Check sheet for the modelled part. Datum: model origin and axes. Units: mm. Give positions to 0.01 mm unless a question says otherwise; leave off trailing zeros. Loops run counter-clockwise (first coordinate to the right, second up) from the corner with the lowest first, then second, coordinate; pieces in that order, holes last. Notation, with made-up numbers: (27.5, 54.5) -> (83.5, 54.5) arc R13 cw to (83.5, 59.5) -> close; hole circle Ø5 at (-36, -25.75). An arc over 180 degrees is marked (long way). Write each question's results on one line, items separated by ' | '. Start each with the question number.
Item 1: Cross-section at B-B on z = 1.4. Enter the section's corners in (x, y).
Item 2: Cross-section at C-C on x = -15. Enter the section's corners in (y, z).
Item 3: Cross-section at A-A on y = 19.5. Enter the section's corners in (x, z), then the cut area to 3 significant figures.
Item 4: Scan lines: line 1 along X through (y, z) = (-7, 0.65); line 2 along Y through (x, z) = (2, 1.7); line 3 along X through (y, z) = (7.5, 2.25). Record each from-to range of solid material in increasing order.
from build123d import *

# Parameters (mm, degrees)
SKETCH1_W           = 40
SKETCH1_H           = 50
SKETCH1_W_2         = 10
SKETCH1_H_2         = 3
BOSS_EXTRUDE1_DEPTH = 3


with BuildPart() as part:
    # Sketch1 → Boss-Extrude1 (new body)
    with BuildSketch(Plane.XY):
        Rectangle(SKETCH1_W, SKETCH1_H)
        with Locations((0, 19.992227475)):
            Rectangle(SKETCH1_W_2, SKETCH1_H_2, mode=Mode.SUBTRACT)
        with Locations((0, 6.878051322)):
            Rectangle(SKETCH1_W_2, SKETCH1_H_2, mode=Mode.SUBTRACT)
        with BuildLine():
            Line((-12.5, -3.7753024), (-12.5, -21.394229107))
            ThreePointArc((-12.5, -21.394229107), (-15, -23.894229107), (-17.5, -21.394229107))
            Line((-17.5, -21.394229107), (-17.5, -3.7753024))
            ThreePointArc((-17.5, -3.7753024), (-15, -1.2753024), (-12.5, -3.7753024))
        make_face(mode=Mode.SUBTRACT)
        with BuildLine():
            Line((12.5, -3.7753024), (12.5, -21.394229107))
            ThreePointArc((12.5, -21.394229107), (15, -23.894229107), (17.5, -21.394229107))
            Line((17.5, -21.394229107), (17.5, -3.7753024))
            ThreePointArc((17.5, -3.7753024), (15, -1.2753024), (12.5, -3.7753024))
        make_face(mode=Mode.SUBTRACT)
    extrude(amount=BOSS_EXTRUDE1_DEPTH)


solid = part.part
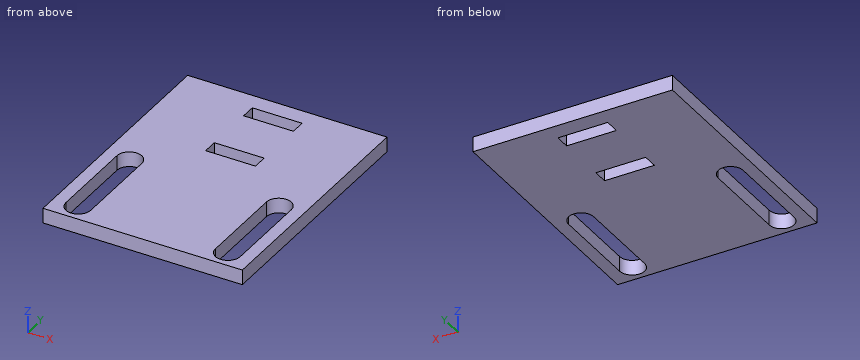
Answer sheet:
1) outline: (-20, -25) -> (20, -25) -> (20, 25) -> (-20, 25) -> close; hole (-17.5, -21.39) arc R2.5 ccw to (-12.5, -21.39) -> (-12.5, -3.78) arc R2.5 ccw to (-17.5, -3.78) -> close; hole (-5, 5.38) -> (5, 5.38) -> (5, 8.38) -> (-5, 8.38) -> close; hole (-5, 18.49) -> (5, 18.49) -> (5, 21.49) -> (-5, 21.49) -> close; hole (12.5, -21.39) arc R2.5 ccw to (17.5, -21.39) -> (17.5, -3.78) arc R2.5 ccw to (12.5, -3.78) -> close
2) outline: (-25, 0) -> (-23.89, 0) -> (-23.89, 3) -> (-25, 3) -> close; (-1.28, 0) -> (25, 0) -> (25, 3) -> (-1.28, 3) -> close
3) outline: (-20, 0) -> (-5, 0) -> (-5, 3) -> (-20, 3) -> close; (5, 0) -> (20, 0) -> (20, 3) -> (5, 3) -> close | area: 90.0 mm²
4) line 1: x = -20 to -17.5, -12.5 to 12.5, 17.5 to 20 | line 2: y = -25 to 5.38, 8.38 to 18.49, 21.49 to 25 | line 3: x = -20 to -5, 5 to 20
